The model under review builds one solid part; all positions refer to its coordinate system, in mm. A direction names the side the tool comes from. Round coordinates to 2 decimals unless told otherwise and drop trailing zeros. Write each loop counter-clockwise with the first axis right and the second up, starting at its lowest first coordinate (ties: lowest second). Pieces come first, ordered by that corner, then holes. Notation, with made-up numbers: (71.25, 37) - (118.25, 37) arc R16 cw to (118.25, 55) - close; hole circle Ø6 at (-27, 66.25). An arc over 180 degrees is marked (long way). Write each question's results on one line, items separated by ' | '.
```python
from build123d import *

# Parameters (mm, degrees)
SKETCH_1_W               = 79
SKETCH_1_H               = 57
SKETCH_1_W_2             = 71
SKETCH_1_H_2             = 49
SKETCH_1_R               = 1.5
EXTRUDE_1_DEPTH          = 2
SKETCH_2_W               = 79
SKETCH_2_H               = 2
EXTRUDE_2_DEPTH          = 32
CUT_EXTRUDE_1_DEPTH      = 1
CUT_EXTRUDE_1_DEPTH_BACK = 62.719121834
SKETCH_3_W               = 1
SKETCH_3_H               = 55
CUT_EXTRUDE_2_DEPTH      = 37.5
CUT_EXTRUDE_2_DEPTH_BACK = 62.719121834
SKETCH_4_W               = 1
SKETCH_4_H               = 1
EXTRUDE_3_DEPTH          = 2
EXTRUDE_3_DEPTH_BACK     = 32
SKETCH_5_W               = 53.5
SKETCH_5_H               = 2
SKETCH_5_W_2             = 19.5


with BuildPart() as part:
    # 草图1 → 凸台-拉伸1 (new body)
    # profile 1 of 4: a face of its own
    with BuildSketch(Plane(origin=(0, 0, 0), x_dir=(1, 0, 0), z_dir=(0, 1, 0))):
        Rectangle(SKETCH_1_W, SKETCH_1_H)
        Rectangle(SKETCH_1_W_2, SKETCH_1_H_2, mode=Mode.SUBTRACT)
    # profile 2 of 4: a face of its own
    with BuildSketch(Plane(origin=(0, 0, 0), x_dir=(1, 0, 0), z_dir=(0, 1, 0))):
        Rectangle(SKETCH_1_W_2, SKETCH_1_H_2)
    # profile 3 of 4: a face of its own
    with BuildSketch(Plane(origin=(0, 0, 0), x_dir=(1, 0, 0), z_dir=(0, 1, 0))):
        with BuildLine():
            Line((20, -28.5), (14, -28.5))
            Line((14, -28.5), (14, -32))
            ThreePointArc((14, -32), (17, -35), (20, -32))
            Line((20, -32), (20, -28.5))
        make_face()
        with Locations(Location((17, -32, 0), (0, 0, 270))):
            Circle(SKETCH_1_R, mode=Mode.SUBTRACT)
    # profile 4 of 4: a face of its own
    with BuildSketch(Plane(origin=(0, 0, 0), x_dir=(1, 0, 0), z_dir=(0, 1, 0))):
        with BuildLine():
            Line((14, 32), (14, 28.5))
            Line((14, 28.5), (20, 28.5))
            Line((20, 28.5), (20, 32))
            ThreePointArc((20, 32), (17, 35), (14, 32))
        make_face()
        with Locations(Location((17, 32, 0), (0, 0, 270))):
            Circle(SKETCH_1_R, mode=Mode.SUBTRACT)
    extrude(amount=EXTRUDE_1_DEPTH)

    # 草图2 → 凸台-拉伸2 (add)
    with BuildSketch(Plane(origin=(0, 0, 0), x_dir=(1, 0, 0), z_dir=(0, 1, 0))):
        with Locations((0, 27.5)):
            Rectangle(SKETCH_2_W, SKETCH_2_H)
        with Locations((0, -27.5)):
            Rectangle(SKETCH_2_W, SKETCH_2_H)
    extrude(amount=-EXTRUDE_2_DEPTH)

    # 草图3 → 切除-拉伸1 (cut, two sides: drawn at the far end of the back side and taken through both)
    with BuildSketch(Plane(origin=(0, 0, 0), x_dir=(1, 0, 0), z_dir=(0, 1, 0)).offset(-CUT_EXTRUDE_1_DEPTH_BACK)):
        with Locations((38, 0)):
            Rectangle(SKETCH_3_W, SKETCH_3_H)
    extrude(amount=CUT_EXTRUDE_1_DEPTH + CUT_EXTRUDE_1_DEPTH_BACK, mode=Mode.SUBTRACT)

    # 草图4 → 切除-拉伸2 (cut, two sides: drawn at the far end of the back side and taken through both)
    with BuildSketch(Plane(origin=(0, 0, 0), x_dir=(0, 0, -1), z_dir=(1, 0, 0)).offset(-CUT_EXTRUDE_2_DEPTH_BACK)):
        with Locations((-27, -30.5)):
            Rectangle(SKETCH_4_W, SKETCH_4_H)
        with Locations((27, -30.5)):
            Rectangle(SKETCH_4_W, SKETCH_4_H)
    extrude(amount=CUT_EXTRUDE_2_DEPTH + CUT_EXTRUDE_2_DEPTH_BACK, mode=Mode.SUBTRACT)

    # 草图5 → 凸台-拉伸3 (add, two sides: drawn at the far end of the back side and taken through both)
    with BuildSketch(Plane(origin=(0, 0, 0), x_dir=(1, 0, 0), z_dir=(0, 1, 0)).offset(-EXTRUDE_3_DEPTH_BACK)):
        with Locations((-12.75, 29.5)):
            Rectangle(SKETCH_5_W, SKETCH_5_H)
        with Locations((-12.75, -29.5)):
            Rectangle(SKETCH_5_W, SKETCH_5_H)
        with Locations((29.75, 29.5)):
            Rectangle(SKETCH_5_W_2, SKETCH_5_H)
        with Locations((29.75, -29.5)):
            Rectangle(SKETCH_5_W_2, SKETCH_5_H)
    extrude(amount=EXTRUDE_3_DEPTH + EXTRUDE_3_DEPTH_BACK)


solid = part.part
```
Q1. We need section A-A (y = -6). State the section outline as (x, z) points, plus the area to 3 significant figures.
Evaluation:
outline: (-39.5, -30.5) - (14, -30.5) - (14, -28.5) - (20, -28.5) - (20, -30.5) - (39.5, -30.5) - (39.5, -26.5) - (38.5, -26.5) - (38.5, -27.5) - (37.5, -27.5) - (37.5, -26.5) - (-39.5, -26.5) - close; (-39.5, 26.5) - (37.5, 26.5) - (37.5, 27.5) - (38.5, 27.5) - (38.5, 26.5) - (39.5, 26.5) - (39.5, 30.5) - (20, 30.5) - (20, 28.5) - (14, 28.5) - (14, 30.5) - (-39.5, 30.5) - close | area: 606 mm^2
Q2. Tool access review of faces 1 (the flat face through (17, 0, -30)), 2 (the flat face through (-2, 0, 0)), 3 (the cylindrical face through (17, 1, 35)), 4 (the flat face through (38.5, 0.3, 12.4)), 5 (the flat face through (17, -16, 28.5)): name each direction out of +Z, -Z, +X, -X, +Y, -Y from which nothing blocks a thin tool from reaching the whole face with its end or side.
Evaluation:
face 1: -Z, -Y | face 2: +X, -X, -Y | face 3: +Z, +Y, -Y | face 4: -Y | face 5: +Z, -Y
Q3. We need section B-B (x = 17). State the section outline as (y, z) points, plus the area to 3 significant figures.
Evaluation:
outline: (-32, -28.5) - (0, -28.5) - (0, -30.5) - (2, -30.5) - (2, 30.5) - (0, 30.5) - (0, 28.5) - (-32, 28.5) - (-32, 26.5) - (-31, 26.5) - (-31, 27.5) - (-30, 27.5) - (-30, 26.5) - (0, 26.5) - (0, -26.5) - (-30, -26.5) - (-30, -27.5) - (-31, -27.5) - (-31, -26.5) - (-32, -26.5) - close; (0, -35) - (2, -35) - (2, -33.5) - (0, -33.5) - close; (0, 33.5) - (2, 33.5) - (2, 35) - (0, 35) - close | area: 254 mm^2
Q4. We need section C-C (z = 14). State the section outline as (x, y) points, plus the area to 3 significant figures.
Evaluation:
outline: (-39.5, 0) - (37.5, 0) - (37.5, 1) - (38.5, 1) - (38.5, 0) - (39.5, 0) - (39.5, 2) - (-39.5, 2) - close | area: 157 mm^2
Q5. For probe 1 along X at (y, z) = (-19, 27); probe 2 along Z at (x, y) = (7, -27); probe 3 along X at (y, z) = (1, -32), list the stretches that pass through material, from the lowest coordinate up.
Evaluation:
probe 1: x = -39.5 to 37.5, 38.5 to 39.5 | probe 2: z = -30.5 to -26.5, 26.5 to 30.5 | probe 3: x = 14 to 15.5, 18.5 to 20
Q6. The part is to be moulded in two halves that separate along X. For faces 6 (the flat face through (20, -16, -29)), 7 (the flat face through (-39.5, 1, 5)), 8 (the flat face through (-2, -15, 26.5)), say which applies: released by +X, released by -X, zero draft, split by the parting line, or undercut.
Evaluation:
face 6: undercut | face 7: released by -X | face 8: zero draft
Q7. Insertion check: P1, Ø10, axis at x = -3.5, y = -23, coming from the -Z side; P2, Ø3, axis at x = -10.5, z = -19.5, coming from the -Y side; P3, Ø1.8, axis at x = 17.5, y = -18.5, coming from the +Z side. Each pin has a flat end and moves straight along its axis. Give the tip position at first contact, or say it passes through.
Evaluation:
P1: stops at z = -30.5 | P2: stops at y = 0 | P3: stops at z = 28.5
Q8. We need section D-D (x = 29). State the section outline as (y, z) points.
Evaluation:
outline: (-32, -30.5) - (2, -30.5) - (2, 30.5) - (-32, 30.5) - (-32, 26.5) - (-31, 26.5) - (-31, 27.5) - (-30, 27.5) - (-30, 26.5) - (0, 26.5) - (0, -26.5) - (-30, -26.5) - (-30, -27.5) - (-31, -27.5) - (-31, -26.5) - (-32, -26.5) - close
